The listing builds one solid part. Answer for the finished solid, in the listing's coordinates (mm). Give positions to 0.01 mm unless a question says otherwise; leave off trailing zeros. Loops run counter-clockwise (first coordinate to the right, second up) from the corner with the lowest first, then second, coordinate; pieces in that order, holes last.
Item 1: Section C-C, the plane y = -5 is taken. Give the number of separate pieces and of enclosed holes in the cut face, and give its area (3 significant figures).
Item 2: Section B-B, the plane x = 0 is taken. Give the vertices of the cut face in (y, z), and give its area (3 significant figures).
Item 3: Consider line 1 along X through (y, z) = (-0.75, -9.5); line 2 along X through (y, z) = (-4.25, -28); line 3 along X through (y, z) = (-4, -59.5). Determine where each line is inside the solid, lowest interval first.
Item 4: Section D-D, the plane z = -25.5 is taken. Give the vertices of the cut face in (x, y).
Item 5: Each of these flat-tipped pins is pushed along its axis until it touches: pin 1 Ø5 at (x, z) = (-15.72, -28.73) entering from +Y; pin 2 Ø2 at (x, y) = (27.5, -5.5) entering from -Z; pin 3 Ø1.5 at (y, z) = (-0.5, -71) entering from -X; pin 4 Ø1 at (y, z) = (-3.5, -12.5) entering from -X. Where does it stop, or does it pass through?
Item 6: Section A-A, the plane z = -44.45 is taken. Give the vertices of the cut face in (x, y).
from build123d import *

# Parameters (mm, degrees)
BOSS_EXTRUDE1_DEPTH       = 6.35
F_6_CLEARANCE_HOLE1_D     = 3.7973
FILLET1_R                 = 17.78
F_7_16_20_TAPPED_HOLE1_D  = 9.92124
F_6_CLEARANCE_HOLE2_D     = 3.7973
F_6_CLEARANCE_HOLE2_DEPTH = 6.35
CUT_EXTRUDE1_DEPTH        = 7.35
FILLET2_R                 = 25.4


with BuildPart() as part:
    # Sketch1 → Boss-Extrude1 (new body)
    with BuildSketch(Plane(origin=(0, 0, 0), x_dir=(1, 0, 0), z_dir=(0, 1, 0))):
        Polygon((-57.15, 0), (0, 114.3), (57.15, 0), align=None)
    extrude(amount=-BOSS_EXTRUDE1_DEPTH)

    # #6 Clearance Hole1 (through all)
    with Locations(Plane(origin=(0, 0, 0), x_dir=(1, 0, 0), z_dir=(0, 1, 0))):
        with Locations((28.575, 9.525), (9.525, 9.525), (-9.525, 79.375), (9.525, 79.375), (-28.575, 9.525), (-9.525, 9.525)):
            Hole(F_6_CLEARANCE_HOLE1_D / 2)

    # Fillet1
    fillet1_edges = [part.edges().sort_by_distance(p)[0] for p in [
        (-57.15, -3.175, 0),
        (0, -3.175, -114.3),
        (57.15, -3.175, 0),
    ]]
    fillet(fillet1_edges, radius=FILLET1_R)

    # 7/16-20 Tapped Hole1 (through all)
    with Locations(Plane(origin=(0, 0, 0), x_dir=(1, 0, 0), z_dir=(0, 1, 0))):
        with Locations((0, 44.45)):
            Hole(F_7_16_20_TAPPED_HOLE1_D / 2)

    # #6 Clearance Hole2
    with Locations(Plane(origin=(0, 0, 0), x_dir=(1, 0, 0), z_dir=(0, 1, 0))):
        with Locations((-15.715448212, 60.165448212), (15.715448212, 28.734551788), (-15.715448212, 28.734551788), (15.715448212, 60.165448212)):
            Hole(F_6_CLEARANCE_HOLE2_D / 2, depth=F_6_CLEARANCE_HOLE2_DEPTH)

    # Sketch9 → Cut-Extrude1 (cut, through all)
    with BuildSketch(Plane(origin=(0, 0, 0), x_dir=(1, 0, 0), z_dir=(0, 1, 0))):
        with BuildLine():
            ThreePointArc((15.902915456, 82.494169088), (0, 92.32271136), (-15.902915456, 82.494169088))
            Line((-15.902915456, 82.494169088), (-44.284271136, 25.731457728))
            ThreePointArc((-44.284271136, 25.731457728), (-43.505927053, 8.432500827), (-28.38135568, 0))
            Line((-28.38135568, 0), (28.38135568, 0))
            ThreePointArc((28.38135568, 0), (43.505927053, 8.432500827), (44.284271136, 25.731457728))
            Line((44.284271136, 25.731457728), (15.902915456, 82.494169088))
        make_face()
        with BuildLine():
            Line((-22.376598212, 60.165448212), (-22.376598212, 61.212248927))
            Line((-22.376598212, 61.212248927), (-22.055517914, 62.208591744))
            Line((-22.055517914, 62.208591744), (-15.865069677, 81.41814361))
            ThreePointArc((-15.865069677, 81.41814361), (-13.446812927, 84.759264359), (-9.525, 86.03615))
            Line((-9.525, 86.03615), (9.525, 86.03615))
            ThreePointArc((9.525, 86.03615), (13.446812927, 84.759264359), (15.865069677, 81.41814361))
            Line((15.865069677, 81.41814361), (22.055518291, 62.208590573))
            Line((22.055518291, 62.208590573), (22.376598212, 61.212248927))
            Line((22.376598212, 61.212248927), (22.376598212, 60.165448212))
            Line((22.376598212, 60.165448212), (22.376598212, 30.758347904))
            Line((22.376598212, 30.758347904), (34.110328487, 13.230544207))
            ThreePointArc((34.110328487, 13.230544207), (34.948483062, 11.461396908), (35.23615, 9.525))
            ThreePointArc((35.23615, 9.525), (33.285144336, 4.814855664), (28.575, 2.86385))
            Line((28.575, 2.86385), (9.525000022, 2.86385))
            Line((9.525000022, 2.86385), (-9.525, 2.86385))
            Line((-9.525, 2.86385), (-28.575, 2.86385))
            ThreePointArc((-28.575, 2.86385), (-34.450972478, 6.387506292), (-34.110328487, 13.230544207))
            Line((-34.110328487, 13.230544207), (-22.376598212, 30.758347904))
            Line((-22.376598212, 30.758347904), (-22.376598212, 60.165448212))
        make_face(mode=Mode.SUBTRACT)
    extrude(amount=-CUT_EXTRUDE1_DEPTH, mode=Mode.SUBTRACT)

    # Fillet2
    fillet2_edges = [part.edges().sort_by_distance(p)[0] for p in [
        (22.376598212, -3.175, -30.758347904),
        (22.376598212, -3.175, -61.212248927),
        (-22.376598212, -3.175, -61.212248927),
        (-22.376598212, -3.175, -30.758347904),
    ]]
    fillet(fillet2_edges, radius=FILLET2_R)


solid = part.part
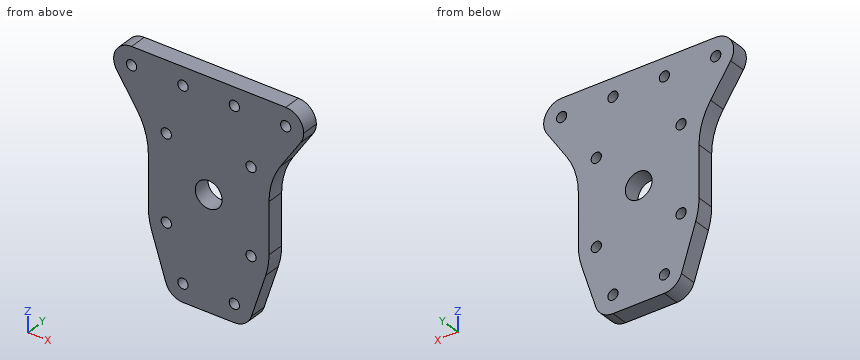
Worked answers:
1. separate pieces: 1
1. enclosed holes: 11
1. area: 3,780 mm2
2. outline: (-6.35, -86.04) - (0, -86.04) - (0, -49.41) - (-6.35, -49.41) - close; (-6.35, -39.49) - (0, -39.49) - (0, -2.86) - (-6.35, -2.86) - close
2. area: 465 mm2
3. line 1: x = -35.24 to -30.47, -26.68 to -11.42, -7.63 to 7.63, 11.42 to 26.68, 30.47 to 35.24
3. line 2: x = -24.64 to -17.47, -13.96 to 13.96, 17.47 to 24.64
3. line 3: x = -22.27 to -17.49, -13.94 to 13.94, 17.49 to 22.27
4. outline: (-25.94, -6.35) - (25.94, -6.35) - (25.94, 0) - (-25.94, 0) - close
5. pin 1: stops at y = 0
5. pin 2: stops at z = -24.6
5. pin 3: stops at x = -19.46
5. pin 4: stops at x = -34.76
6. outline: (-22.38, -6.35) - (-4.96, -6.35) - (-4.96, 0) - (-22.38, 0) - close; (4.96, -6.35) - (22.38, -6.35) - (22.38, 0) - (4.96, 0) - close
